For this review, take the finished solid that the model builds, in its own axes (mm). Round coordinates to 2 decimals unless told otherwise and drop trailing zeros. Loops run counter-clockwise (first coordinate to the right, second up) from the corner with the lowest first, then second, coordinate; pieces in that order, holes last. Notation, with made-up numbers: (41, 46.25) -> (60, 46.25) arc R16 cw to (60, 71.25) -> close; hole circle Ø5 at (4, 84.5). An arc over 180 degrees is marked (long way). Write each question's results on one line, items separated by ' | '.
```python
from build123d import *

# Parameters (mm, degrees)
BOSS_EXTRUDE2_DEPTH = 25.4
SKETCH2_R           = 3.571875
CUT_EXTRUDE1_DEPTH  = 25.4


with BuildPart() as part:
    # Sketch1 → Boss-Extrude2 (new body)
    # profile 1 of 4: a face of its own
    with BuildSketch(Plane(origin=(0, 0, 0), x_dir=(1, 0, 0), z_dir=(0, 1, 0))):
        Polygon((-69.664713837, 334.281849575), (-324.328930675, -106.809512857), (-254.664216837, -227.472336718), (254.664216837, -227.472336718), (324.328930675, -106.809512857), (69.664713837, 334.281849575), align=None)
        Polygon((-239.99952, -202.072336718), (-294.999537, -106.809512857), (-55.000017, 308.881849575), (55.000017, 308.881849575), (294.999537, -106.809512857), (239.99952, -202.072336718), align=None, mode=Mode.SUBTRACT)
    # profile 2 of 4: a face of its own
    with BuildSketch(Plane(origin=(0, 0, 0), x_dir=(1, 0, 0), z_dir=(0, 1, 0))):
        Polygon((-93.352551626, -202.072336718), (-221.676052813, 20.190487143), (-251.005446488, -30.609512857), (-152.011338976, -202.072336718), align=None)
    # profile 3 of 4: a face of its own
    with BuildSketch(Plane(origin=(0, 0, 0), x_dir=(1, 0, 0), z_dir=(0, 1, 0))):
        Polygon((251.005446488, -30.609512857), (221.676052813, 20.190487143), (93.352551626, -202.072336718), (152.011338976, -202.072336718), align=None)
    # profile 4 of 4: a face of its own
    with BuildSketch(Plane(origin=(0, 0, 0), x_dir=(1, 0, 0), z_dir=(0, 1, 0))):
        Polygon((98.994107512, 232.681849575), (-98.994107512, 232.681849575), (-128.323501187, 181.881849575), (128.323501187, 181.881849575), align=None)
    extrude(amount=BOSS_EXTRUDE2_DEPTH)

    # Sketch2 → Cut-Extrude1 (cut)
    with BuildSketch(Plane.XZ):
        with Locations(Location((-289.610551128, 141.543510188, 0), (0, 0, 270))):
            Circle(SKETCH2_R)
        with Locations(Location((-267.385551128, 180.038339387, 0), (0, 0, 270))):
            Circle(SKETCH2_R)
        with Locations(Location((267.385551128, 180.038339387, 0), (0, 0, 270))):
            Circle(SKETCH2_R)
        with Locations(Location((289.610551128, 141.543510188, 0), (0, 0, 270))):
            Circle(SKETCH2_R)
        with Locations(Location((22.225, -321.581849575, 0), (0, 0, 270))):
            Circle(SKETCH2_R)
        with Locations(Location((-22.225, -321.581849575, 0), (0, 0, 270))):
            Circle(SKETCH2_R)
        with Locations(Location((-201.622370104, 90.743510188, 0), (0, 0, 270))):
            Circle(SKETCH2_R)
        with Locations(Location((-179.397370104, 129.238339387, 0), (0, 0, 270))):
            Circle(SKETCH2_R)
        with Locations(Location((-157.400324847, 116.538339387, 0), (0, 0, 270))):
            Circle(SKETCH2_R)
        with Locations(Location((-179.625324847, 78.043510188, 0), (0, 0, 270))):
            Circle(SKETCH2_R)
        with Locations(Location((201.622370104, 90.743510188, 0), (0, 0, 270))):
            Circle(SKETCH2_R)
        with Locations(Location((179.397370104, 129.238339387, 0), (0, 0, 270))):
            Circle(SKETCH2_R)
        with Locations(Location((-22.225, -219.981849575, 0), (0, 0, 270))):
            Circle(SKETCH2_R)
        with Locations(Location((22.225, -219.981849575, 0), (0, 0, 270))):
            Circle(SKETCH2_R)
        with Locations(Location((179.625324847, 78.043510188, 0), (0, 0, 270))):
            Circle(SKETCH2_R)
        with Locations(Location((157.400324847, 116.538339387, 0), (0, 0, 270))):
            Circle(SKETCH2_R)
        with Locations(Location((-22.225, -194.581849575, 0), (0, 0, 270))):
            Circle(SKETCH2_R)
        with Locations(Location((22.225, -194.581849575, 0), (0, 0, 270))):
            Circle(SKETCH2_R)
    extrude(amount=-CUT_EXTRUDE1_DEPTH, mode=Mode.SUBTRACT)


solid = part.part
```
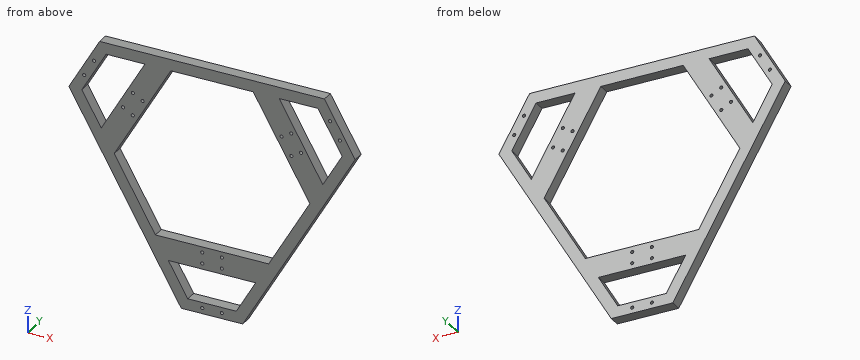
1. Consider section B-B (z = 66). State the section outline as (x, y) points.
Values found:
outline: (-300.77, 0) -> (-271.44, 0) -> (-271.44, 25.4) -> (-300.77, 25.4) -> close; (-230.57, 0) -> (-171.91, 0) -> (-171.91, 25.4) -> (-230.57, 25.4) -> close; (171.91, 0) -> (230.57, 0) -> (230.57, 25.4) -> (171.91, 25.4) -> close; (271.44, 0) -> (300.77, 0) -> (300.77, 25.4) -> (271.44, 25.4) -> close
2. Consider section D-D (z = -250.5). State the section outline as (x, y) points, plus the area to 3 significant figures.
Values found:
outline: (-118.04, 0) -> (-88.71, 0) -> (-88.71, 25.4) -> (-118.04, 25.4) -> close; (88.71, 0) -> (118.04, 0) -> (118.04, 25.4) -> (88.71, 25.4) -> close | area: 1,490 mm2
3. For pin 1 (12.5 mm diameter, centred on x = -207.5, y = 18.5, fed in from -Z); pin 2 (6 mm diameter, centred on y = 16.5, z = 121, fed in from +X); pin 3 (3 mm diameter, centred on x = 123.5, y = 16, fed in from -Z), all flat-tipped, find the tip position at first contact; note any pin that passes through.
Values found:
pin 1: stops at z = -106.37 | pin 2: stops at x = 317.87 | pin 3: stops at z = -243.63
4. To check wall thickness, follow probe 1 along Z at (x, y) = (5, 4.75); probe 2 along Z at (x, y) = (-270.5, 23.75); probe 3 along X at (y, z) = (9.75, 132.5). State the ranges of each line that lie inside material, in increasing order.
Values found:
probe 1: z = -334.28 to -308.88, -232.68 to -181.88, 202.07 to 227.47 | probe 2: z = 13.58 to 64.38, 149.24 to 178.29, 181.79 to 200.04 | probe 3: x = -309.5 to -280.17, -192.18 to -180.85, -177.94 to -133.52, 133.52 to 177.94, 180.85 to 192.18, 280.17 to 309.5
5. Consider section A-A (x = -39.5). State the section outline as (y, z) points.
Values found:
outline: (0, -334.28) -> (25.4, -334.28) -> (25.4, -308.88) -> (0, -308.88) -> close; (0, -232.68) -> (25.4, -232.68) -> (25.4, -181.88) -> (0, -181.88) -> close; (0, 202.07) -> (25.4, 202.07) -> (25.4, 227.47) -> (0, 227.47) -> close
6. Consider section C-C (x = -107.5). State the section outline as (y, z) points, plus the area to 3 significant figures.
Values found:
outline: (0, -268.75) -> (25.4, -268.75) -> (25.4, -181.88) -> (0, -181.88) -> close; (0, 177.57) -> (25.4, 177.57) -> (25.4, 227.47) -> (0, 227.47) -> close | area: 3,470 mm2
